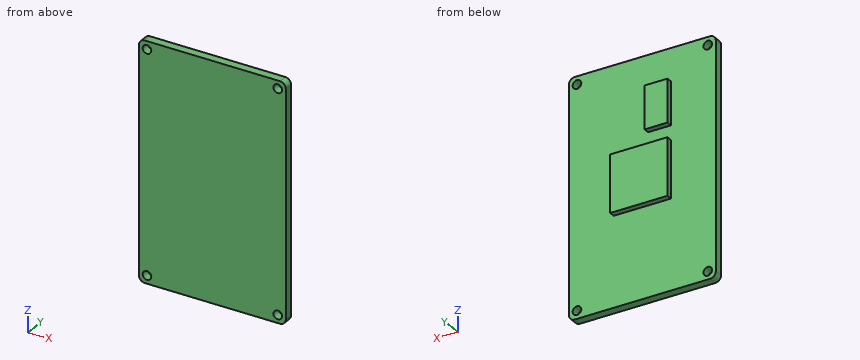
```python
from build123d import *

# Parameters (mm, degrees)
SKETCH_1_W      = 51.24
SKETCH_1_H      = 82.8
SKETCH_1_R      = 1.5
EXTRUDE_1_DEPTH = 3
SKETCH_2_W      = 20
SKETCH_2_H      = 20
SKETCH_2_W_2    = 8
SKETCH_2_H_2    = 15
EXTRUDE_2_DEPTH = 2
FILLET_1_R      = 2


with BuildPart() as part:
    # 草图1 → 凸台-拉伸1 (new body)
    with BuildSketch(Plane(origin=(0, 0, 0), x_dir=(1, 0, 0), z_dir=(0, 1, 0))):
        Rectangle(SKETCH_1_W, SKETCH_1_H)
        with Locations(Location((22.82, 38.6, 0), (0, 0, 270))):
            Circle(SKETCH_1_R, mode=Mode.SUBTRACT)
        with Locations(Location((-22.82, 38.6, 0), (0, 0, 90))):
            Circle(SKETCH_1_R, mode=Mode.SUBTRACT)
        with Locations(Location((-22.82, -38.6, 0), (0, 0, 270))):
            Circle(SKETCH_1_R, mode=Mode.SUBTRACT)
        with Locations(Location((22.82, -38.6, 0), (0, 0, 90))):
            Circle(SKETCH_1_R, mode=Mode.SUBTRACT)
    extrude(amount=EXTRUDE_1_DEPTH)

    # 草图2 → 凸台-拉伸2 (add)
    with BuildSketch(Plane(origin=(0, 3, 0), x_dir=(1, 0, 0), z_dir=(0, 1, 0))):
        Rectangle(SKETCH_2_W, SKETCH_2_H)
        with Locations((-6, -22.5)):
            Rectangle(SKETCH_2_W_2, SKETCH_2_H_2)
    extrude(amount=EXTRUDE_2_DEPTH)

    # 圆角1
    fillet_1_edges = [part.edges().sort_by_distance(p)[0] for p in [
        (-25.62, 1.5, 41.4),
        (-25.62, 1.5, -41.4),
        (25.62, 1.5, -41.4),
        (25.62, 1.5, 41.4),
    ]]
    fillet(fillet_1_edges, radius=FILLET_1_R)


solid = part.part
```
Input: part model. Units: mm. Frame: model coordinates. Round coordinates to 2 decimals unless told otherwise and drop trailing zeros. Write each loop counter-clockwise with the first axis right and the second up, starting at its lowest first coordinate (ties: lowest second). Pieces come first, ordered by that corner, then holes. Notation, with made-up numbers: (62, 11) -> (79, 11) arc R22 ccw to (79, 42) -> close; hole circle Ø8 at (-36, -9). An arc over 180 degrees is marked (long way). Answer as CSV lines item,"result".
1. Section A-A (z = 38.6). Return the cut outline in (x, y).
Geometry says:
outline,"(-25.62, 0) -> (-24.32, 0) -> (-24.32, 3) -> (-25.62, 3) -> close; (-21.32, 0) -> (21.32, 0) -> (21.32, 3) -> (-21.32, 3) -> close; (24.32, 0) -> (25.62, 0) -> (25.62, 3) -> (24.32, 3) -> close"
2. Section D-D (x = 3). Return the cut outline in (y, z).
Geometry says:
outline,"(0, -41.4) -> (3, -41.4) -> (3, -10) -> (5, -10) -> (5, 10) -> (3, 10) -> (3, 41.4) -> (0, 41.4) -> close"
3. Section C-C (x = -22.82). Return the cut outline in (y, z).
Geometry says:
outline,"(0, -41.4) -> (3, -41.4) -> (3, -40.1) -> (0, -40.1) -> close; (0, -37.1) -> (3, -37.1) -> (3, 37.1) -> (0, 37.1) -> close; (0, 40.1) -> (3, 40.1) -> (3, 41.4) -> (0, 41.4) -> close"
4. Ray query, L1, parallel to X at y = 1.1, z = -38.6; L2, parallel to Y at x = 23, z = 19; L3, parallel to X at y = 4.85, z = 21. Return the intervals inside material, ascending. Write a range as [from, to].
Geometry says:
L1,"x = [-25.62, -24.32], [-21.32, 21.32], [24.32, 25.62]"
L2,"y = [0, 3]"
L3,"x = [-10, -2]"
5. Section B-B (y = 3.8). Return the cut outline in (x, z).
Geometry says:
outline,"(-10, -10) -> (10, -10) -> (10, 10) -> (-10, 10) -> close; (-10, 15) -> (-2, 15) -> (-2, 30) -> (-10, 30) -> close"
6. Contact query for flat-ended pins moving along their axis: P1, Ø1, axis at y = 4.5, z = 5, coming from the +X side; P2, Ø1.6, axis at y = 4, z = 25, coming from the +X side; P3, Ø1.6, axis at y = 4, z = -0.5, coming from the -X side. Output: stop coordinate, or through.
Geometry says:
P1,"stops at x = 10"
P2,"stops at x = -2"
P3,"stops at x = -10"
